Here's the drawing with two shaded views (mm, measured from the low corner). I have some questions. A direction names the side the tool comes from. Round coordinates to 2 decimals unless told otherwise and drop trailing zeros. Loops run counter-clockwise (first coordinate to the right, second up) from the corner with the lowest first, then second, coordinate; pieces in that order, holes last. Notation, with made-up numbers: (28.5, 60) -> (74.5, 60) arc R24 ccw to (74.5, 76) -> close; hole circle Ø8 at (-27.75, 89.25). An arc over 180 degrees is marked (long way). Write item = value, one per line.
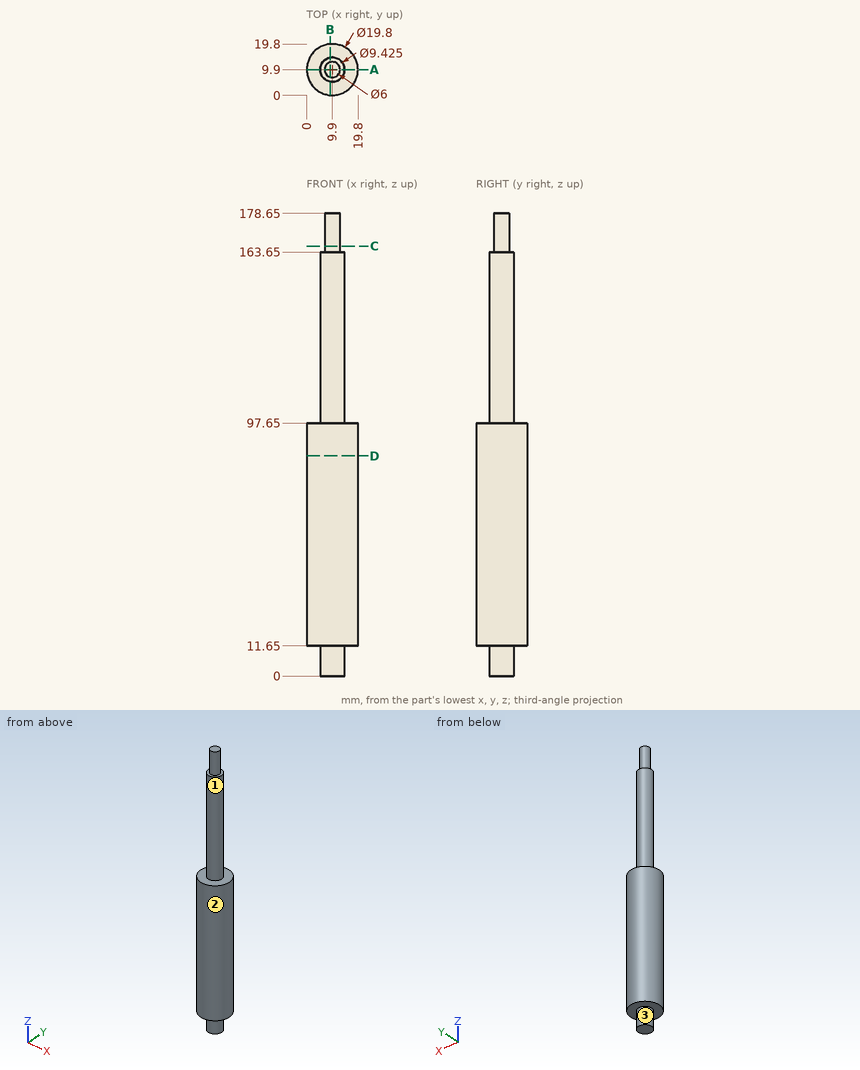
1. Suppose I cut it at B-B, the plane x = 9. List the corners of the cut face in (y, z) for me, and give its area (3 significant figures).
Entries:
outline = (0.04, 11.65) -> (5.27, 11.65) -> (5.27, 0) -> (14.53, 0) -> (14.53, 11.65) -> (19.76, 11.65) -> (19.76, 97.65) -> (14.53, 97.65) -> (14.53, 163.65) -> (12.76, 163.65) -> (12.76, 178.65) -> (7.04, 178.65) -> (7.04, 163.65) -> (5.27, 163.65) -> (5.27, 97.65) -> (0.04, 97.65) -> close
area = 2,500 mm²
2. For the marked faces 1, 2 and 3, which set-ups out of +Z, -Z, +X, -X, +Y, -Y let a thin tool reach every point of the face, with its end or its side?
Entries:
face_1 = +Z
face_2 = +Z, -Z
face_3 = -Z
3. I'm going to push flat-ended pins straight in: pin 1 (10 mm diameter, centred on x = 15.5, y = 5.5, fed in from -Z); pin 2 (4 mm diameter, centred on y = 17, z = 35, fed in from -X); pin 3 (4 mm diameter, centred on x = 15, z = 89.5, fed in from -Y); pin 4 (2 mm diameter, centred on x = 6, z = 97.5, fed in from +Y). Where does each tip first touch, or does it pass through?
Entries:
pin_1 = 0
pin_2 = 1.41
pin_3 = 0.5
pin_4 = 19.37
4. I need wall thicknesses on line 1 (Z direction, x = 13.25, y = 12.5); line 2 (Z direction, x = 8, y = 1.5); line 3 (X direction, y = 14.25, z = 96.5). Which ranges of each line are inside material? Lowest first, please. Write a range as [from, to].
Entries:
line_1 = [0, 163.65]
line_2 = [11.65, 97.65]
line_3 = [1.01, 18.79]
5. Suppose I cut it at A-A, the plane y = 9.9. List the corners of the cut face in (x, z) for me.
Entries:
outline = (0, 11.65) -> (5.19, 11.65) -> (5.19, 0) -> (14.61, 0) -> (14.61, 11.65) -> (19.8, 11.65) -> (19.8, 97.65) -> (14.61, 97.65) -> (14.61, 163.65) -> (12.9, 163.65) -> (12.9, 178.65) -> (6.9, 178.65) -> (6.9, 163.65) -> (5.19, 163.65) -> (5.19, 97.65) -> (0, 97.65) -> close
6. Suppose I cut it at C-C, the plane z = 166. List the corners of the cut face in (x, y) for me.
Entries:
outline = circle Ø6 at (9.9, 9.9)
7. Suppose I cut it at D-D, the plane z = 85. List the corners of the cut face in (x, y) for me, and give its area (3 significant figures).
Entries:
outline = circle Ø19.8 at (9.9, 9.9)
area = 308 mm²
